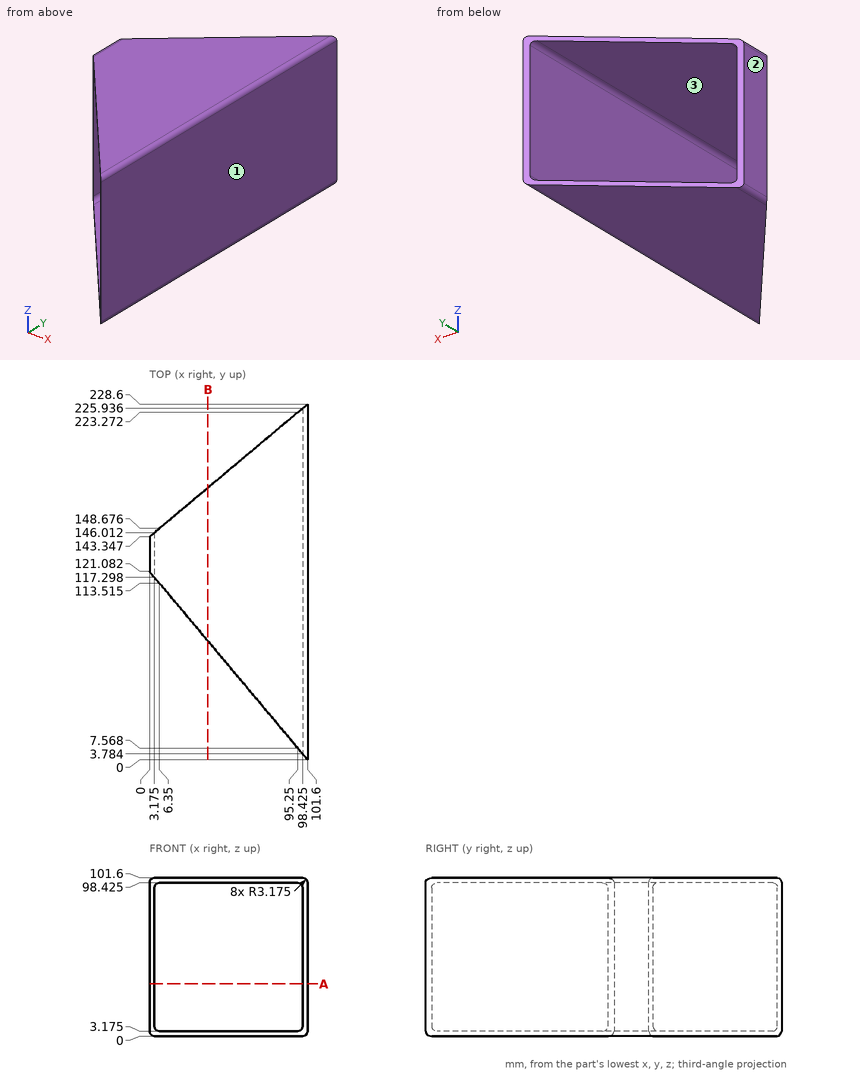
Here's the drawing with two shaded views (mm, measured from the low corner). I have some questions. Coordinates: 2 decimals unless noted, no trailing zeros. Order: outer loops, then holes, each group sorted by start corner. A loop starts at its lowest first (then second) coordinate and runs counter-clockwise, first axis right, second up. Notation, with made-up numbers: (31, -9.5) - (52, -9.5) arc R7 ccw to (52, -1.5) - close; hole circle Ø11 at (19.25, 67.25). An arc over 180 degrees is marked (long way). Answer in a Markdown table with one row per item. Add a question column.
(1) If we mould it in two halves opening along X, with no side actions, what happens to the marked faces 1, 2 and 3? For each: released by +X, released by -X, zero draft, split by the parting line, or undercut.
(2) If we section it at B-B, the plane x = 37.5: Please give me the cut outline in (y, z) (1 decimal), then the cut area to 3 significant figures.
(3) Will this pin go through, and if not, where does the flat tip stop? pin 1 (10 mm diameter, centred on y = 194.5, z = 28, fed in from -X) (3 decimals).
(4) I need wall thicknesses on L1, parallel to Z at x = 71, y = 126 (1 decimal); L2, parallel to X at y = 100.5, z = 39.5 (1 decimal). Which ranges of each line are inside material? Lowest first, please.
(5) If we section it at A-A, the plane z = 33.5: Please give me the cut outline in (x, y) (1 decimal).
Results are:
| question | item | result |
|---|---|---|
| 1 | face 1 | released by +X |
| 1 | face 2 | released by -X |
| 1 | face 3 | undercut |
| 2 | outline | (76.4, 0) - (174.8, 0) - (174.8, 3.2) - (76.4, 3.2) - close; (76.4, 98.4) - (174.8, 98.4) - (174.8, 101.6) - (76.4, 101.6) - close |
| 2 | area | 625 mm2 |
| 3 | pin 1 | stops at x = 98.425 |
| 4 | L1 | z = 0 to 3.2, 98.4 to 101.6 |
| 4 | L2 | x = 98.4 to 101.6 |
| 5 | outline | (0, 121.1) - (3.2, 117.3) - (3.2, 146) - (0, 143.3) - close; (98.4, 3.8) - (101.6, 0) - (101.6, 228.6) - (98.4, 225.9) - close |
